For this review, take the finished solid that the model builds, in its own axes (mm). A direction names the side the tool comes from. Coordinates: 2 decimals unless noted, no trailing zeros. Loops run counter-clockwise (first coordinate to the right, second up) from the corner with the lowest first, then second, coordinate; pieces in that order, holes last. Notation, with made-up numbers: (39.5, 4) -> (67.5, 4) arc R23 ccw to (67.5, 27) -> close; hole circle Ø11 at (-30.75, -29.75). An arc over 180 degrees is marked (long way). Answer in a Markdown table with one row per item.
from build123d import *

# Parameters (mm, degrees)
SKETCH1_W           = 53.34
SKETCH1_H           = 152.4
SKETCH1_R           = 1
BOSS_EXTRUDE1_DEPTH = 6.35
SKETCH2_W           = 32.258
SKETCH2_H           = 6.35
BOSS_EXTRUDE2_DEPTH = 31.75
SKETCH3_W           = 32.258
SKETCH3_H           = 6.35
BOSS_EXTRUDE3_DEPTH = 12.7
CUT_EXTRUDE1_REACH  = 136.322
SKETCH4_R           = 12.573
SKETCH5_W           = 32.258
SKETCH5_H           = 2.671239047
SKETCH5_H_2         = 2.428760953
BOSS_EXTRUDE4_DEPTH = 7.62
FILLET1_R           = 5.08
SKETCH6_W           = 53.34
SKETCH6_H           = 6.35
BOSS_EXTRUDE5_DEPTH = 31.75
CUT_EXTRUDE3_REACH  = 159.154


with BuildPart() as part:
    # Sketch1 → Boss-Extrude1 (new body)
    with BuildSketch(Plane.XY):
        with Locations((-17.091445783, 46.760481928)):
            Rectangle(SKETCH1_W, SKETCH1_H)
        with Locations((-36.141445783, 69.620481928)):
            Circle(SKETCH1_R, mode=Mode.SUBTRACT)
        with Locations((-8.201445783, 69.620481928)):
            Circle(SKETCH1_R, mode=Mode.SUBTRACT)
        with Locations((-41.221445783, 121.690481928)):
            Circle(SKETCH1_R, mode=Mode.SUBTRACT)
        with Locations((7.038554217, 120.420481928)):
            Circle(SKETCH1_R, mode=Mode.SUBTRACT)
    extrude(amount=BOSS_EXTRUDE1_DEPTH)

    # Sketch2 → Boss-Extrude2 (add)
    with BuildSketch(Plane.XY):
        with Locations((-17.091445783, 60.014063864)):
            Rectangle(SKETCH2_W, SKETCH2_H)
    extrude(amount=BOSS_EXTRUDE2_DEPTH)

    # Sketch3 → Boss-Extrude3 (add)
    with BuildSketch(Plane(origin=(0, 63.189063864, 0), x_dir=(1, 0, 0), z_dir=(0, 1, 0))):
        with Locations((-17.091445783, -28.575)):
            Rectangle(SKETCH3_W, SKETCH3_H)
    extrude(amount=BOSS_EXTRUDE3_DEPTH)

    # Sketch4 → Cut-Extrude1 (cut, up to next)
    with BuildSketch(Plane.XY.offset(31.75), mode=Mode.PRIVATE) as cut_extrude1_sk1:
        with Locations((-17.091445783, 78.510481928)):
            Circle(SKETCH4_R)
    cut_extrude1_tool1 = extrude(cut_extrude1_sk1.sketch, amount=-CUT_EXTRUDE1_REACH, mode=Mode.PRIVATE) & part.part
    add(cut_extrude1_tool1.solids().sort_by_distance((-17.091446, 78.510482, 31.75))[0], mode=Mode.SUBTRACT)

    # Sketch5 → Boss-Extrude4 (add)
    with BuildSketch(Plane(origin=(0, 63.189063864, 0), x_dir=(1, 0, 0), z_dir=(0, 1, 0))):
        with Locations((-17.091445783, -26.735619524)):
            Rectangle(SKETCH5_W, SKETCH5_H)
        with Locations((-17.091445783, -30.535619524)):
            Rectangle(SKETCH5_W, SKETCH5_H_2)
    extrude(amount=BOSS_EXTRUDE4_DEPTH)

    # Fillet1
    fillet1_edges = [part.edges().sort_by_distance(p)[0] for p in [
        (-17.091445783, 63.189063864, 25.4),
    ]]
    fillet(fillet1_edges, radius=FILLET1_R)

    # Sketch6 → Boss-Extrude5 (add)
    with BuildSketch(Plane.XY.offset(6.35)):
        with Locations((-17.091445783, -26.264518072)):
            Rectangle(SKETCH6_W, SKETCH6_H)
    extrude(amount=BOSS_EXTRUDE5_DEPTH)

    # Sketch7 → Cut-Extrude3 (cut, up to next)
    with BuildSketch(Plane(origin=(0, -23.089518072, 0), x_dir=(1, 0, 0), z_dir=(0, 1, 0)), mode=Mode.PRIVATE) as cut_extrude3_sk1:
        with BuildLine():
            Line((-36.395445783, -21.844), (2.212554217, -21.844))
            ThreePointArc((2.212554217, -21.844), (5.768554217, -25.4), (2.212554217, -28.956))
            Line((2.212554217, -28.956), (-36.395445783, -28.956))
            ThreePointArc((-36.395445783, -28.956), (-39.951445783, -25.4), (-36.395445783, -21.844))
        make_face()
    cut_extrude3_tool1 = extrude(cut_extrude3_sk1.sketch, amount=-CUT_EXTRUDE3_REACH, mode=Mode.PRIVATE) & part.part
    add(cut_extrude3_tool1.solids().sort_by_distance((-17.091446, -23.089518, 25.4))[0], mode=Mode.SUBTRACT)


solid = part.part
Item 1: For L1, parallel to Y at x = -7, z = 11; L2, parallel to Y at x = -21, z = 30; L3, parallel to Y at x = -13, z = 25.5, list the stretches that pass through material, from the lowest coordinate up.
Worked answers:
| item | result |
|---|---|
| L1 | -29.44 to -23.09, 56.84 to 63.19 |
| L2 | -29.44 to -23.09, 56.84 to 70.81 |
| L3 | 56.84 to 70.81 |
Item 2: Take a section at A-A, the plane x = -20.5. State the section outline as (y, z) points, and give its area (3 significant figures).
Worked answers:
| item | result |
|---|---|
| outline | (-29.44, 0) -> (122.96, 0) -> (122.96, 6.35) -> (63.19, 6.35) -> (63.19, 20.32) arc R5.08 cw to (68.27, 25.4) -> (70.81, 25.4) -> (70.81, 28.07) -> (66.41, 28.07) -> (66.41, 29.32) -> (70.81, 29.32) -> (70.81, 31.75) -> (56.84, 31.75) -> (56.84, 6.35) -> (-23.09, 6.35) -> (-23.09, 21.84) -> (-29.44, 21.84) -> close; (-29.44, 28.96) -> (-23.09, 28.96) -> (-23.09, 38.1) -> (-29.44, 38.1) -> close |
| area | 1,330 mm² |
Item 3: The part is to be moulded in two halves that separate along X. For faces 5 (the flat face through (-17, 64, 31.75)), 6 (the flat face through (-17, 70.809, 27)), 7 (the flat face through (9.579, 35, 6)), say which applies: +X half, -X half, draft (parallel to the pull), parting line (faces both ways), or undercut.
Worked answers:
| item | result |
|---|---|
| face 5 | draft |
| face 6 | undercut |
| face 7 | +X half |
Item 4: Insertion check: pin 1 (1.2 mm diameter, centred on x = -16.5, z = 31, fed in from +Y); pin 2 (8 mm diameter, centred on x = -5, y = 0, fed in from +Z); pin 3 (1.8 mm diameter, centred on x = 7.04, y = 120.42, fed in from -Z); pin 4 (4 mm diameter, centred on x = -2.5, z = 27.5, fed in from +Y). Each pin has a flat end and moves straight along its axis. Give the tip position at first contact, or say it passes through.
Worked answers:
| item | result |
|---|---|
| pin 1 | y = 70.81 |
| pin 2 | z = 6.35 |
| pin 3 | through |
| pin 4 | y = 75.89 |
Item 5: Take a section at B-B, the plane y = 87. State the section outline as (x, z) points, and give its area (3 significant figures).
Worked answers:
| item | result |
|---|---|
| outline | (-43.76, 0) -> (9.58, 0) -> (9.58, 6.35) -> (-43.76, 6.35) -> close |
| area | 339 mm² |
Item 6: For faces 1 (the flat face through (-0.962, 62, 22)), 2 (the flat face through (-17, 69, 29.321)), 3 (the cylindrical face through (5.768, -26.22, 25.322)), 4 (the flat face through (-17, 63.189, 13)), list the 3-axis set-ups (+Z, -Z, +X, -X, +Y, -Y) from which the entire face can be reached by the end or side of a thin tool; tool diameter is ignored.
Worked answers:
| item | result |
|---|---|
| face 1 | +Z, +X, +Y |
| face 2 | +Y |
| face 3 | +Y, -Y |
| face 4 | +X, -X, +Y |
